CAD build for the part. Positions are in the model's coordinates, mm. A direction names the side the tool comes from. Coordinates: 2 decimals unless noted, no trailing zeros. Write each loop counter-clockwise with the first axis right and the second up, starting at its lowest first coordinate (ties: lowest second). Pieces come first, ordered by that corner, then holes. Notation, with made-up numbers: (-35, -36.75) - (0, -36.75) arc R36 ccw to (0, 2.25) - close; hole circle Ø8 at (65, -3). An arc over 180 degrees is marked (long way). Answer in a Markdown table with one row per item. Add a question column.
Q1. Band-saw the part on A-A (x = 0). List the corners of the cut face in (y, z) (3 decimals).
Q2. Two-plate mould, pull along Y, no slides. Class faces 4 (the cylindrical face through (-17.48, 6.86, 18.71)), 5 (the flat face through (18.75, -3, 20)), 6 (the cylindrical face through (-5.158, -3.955, -1.479)): +Y half, -Y half, draft (parallel to the pull), parting line (faces both ways), or undercut.
Q3. Drill centre lines: line 1 along X through (y, z) = (7, 16); line 2 along Z through (x, y) = (5, -8.5); line 3 along Y through (x, z) = (-10, 2.5). Where is each one in solid material? Low to high. Write a range as from..to.
Q4. Pin check, flat tips, straight feed: pin 1 (1 mm diameter, centred on x = -15, z = 16, fed in from +Y); pin 2 (9.5 mm diameter, centred on y = 0, z = 15.25, fed in from +X); pin 3 (0.8 mm diameter, centred on x = -15.5, y = -10.5, fed in from +Z). Stop position of each tip, or through.
Q5. Band-saw the part on C-C (y = -9.5). List the corners of the cut face in (x, z), and give its area (3 significant figures).
Q6. Band-saw the part on B-B (z = 6). List the corners of the cut face in (x, y), and give its area (4 significant figures).
Q7. Band-saw the part on D-D (z = 14.5). List the corners of the cut face in (x, y).
Q8. 3-axis set-ups, long thin cutter, end or side, ignore diameter. For faces 1 (the flat face through (-15.25, -1, 7)), 2 (the flat face through (17, 0, 35)), 3 (the flat face through (16, 6.981, 14)): which of +Z, -Z, +X, -X, +Y, -Y reach the whole face in a straight line?
```python
from build123d import *

# Parameters (mm, degrees)
SKETCH1_W            = 37.5
SKETCH1_H            = 24
SKETCH1_R            = 0.8
SKETCH1_R_2          = 6.5
BOSS_EXTRUDE1_DEPTH  = 3
SKETCH2_W            = 2.5
SKETCH2_H            = 40
BOSS_EXTRUDE2_DEPTH  = 24
BOSS_EXTRUDE3_DEPTH  = 1
BOSS_EXTRUDE4_START  = 31.5
BOSS_EXTRUDE4_DEPTH  = 1
M3_CLEARANCE_HOLE1_D = 3.6
CHAMFER1_SIZE        = 2
SKETCH7_R            = 3
SKETCH7_W            = 11
SKETCH7_H            = 9
CUT_EXTRUDE1_DEPTH   = 57.127087934
FILLET1_R            = 1
BOSS_EXTRUDE5_DEPTH  = 2
BOSS_EXTRUDE6_DEPTH  = 5


with BuildPart() as part:
    # Sketch1 → Boss-Extrude1 (new body)
    with BuildSketch(Plane.XY):
        Rectangle(SKETCH1_W, SKETCH1_H)
        with Locations((0, 9.075)):
            Circle(SKETCH1_R, mode=Mode.SUBTRACT)
        with Locations((7.859180539, -4.5375)):
            Circle(SKETCH1_R, mode=Mode.SUBTRACT)
        with Locations((-7.859180539, -4.5375)):
            Circle(SKETCH1_R, mode=Mode.SUBTRACT)
        Circle(SKETCH1_R_2, mode=Mode.SUBTRACT)
    extrude(amount=-BOSS_EXTRUDE1_DEPTH)

    # Sketch2 → Boss-Extrude2 (add)
    with BuildSketch(Plane(origin=(0, 12, 0), x_dir=(1, 0, 0), z_dir=(0, 1, 0))):
        with Locations((-17.5, -20)):
            Rectangle(SKETCH2_W, SKETCH2_H)
        with Locations((17.5, -20)):
            Rectangle(SKETCH2_W, SKETCH2_H)
    extrude(amount=-BOSS_EXTRUDE2_DEPTH)

    # Sketch4 → Boss-Extrude3 (add)
    with BuildSketch(Plane(origin=(-16.25, 0, 0), x_dir=(0, 0, -1), z_dir=(1, 0, 0))):
        with BuildLine():
            Line((-9.328443352, 3.861127794), (-9.37974654, -3.938739946))
            ThreePointArc((-9.37974654, -3.938739946), (-10.302425145, -6.124404492), (-12.500032536, -7.018265261))
            Line((-12.500032536, -7.018265261), (-15.407950321, -7.018265261))
            Line((-15.407950321, -7.018265261), (-15.407950321, -12))
            Line((-15.407950321, -12), (0, -12))
            Line((0, -12), (0, 12))
            Line((0, 12), (-15.407950321, 12))
            Line((-15.407950321, 12), (-15.407950321, 6.981431896))
            Line((-15.407950321, 6.981431896), (-12.407950321, 6.981431896))
            ThreePointArc((-12.407950321, 6.981431896), (-10.222291202, 6.058740436), (-9.328443352, 3.861127794))
        make_face()
    extrude(amount=BOSS_EXTRUDE3_DEPTH)

    # Sketch4<2> → Boss-Extrude4 (add)
    with BuildSketch(Plane(origin=(-16.25, 0, 0), x_dir=(0, 0, -1), z_dir=(1, 0, 0)).offset(BOSS_EXTRUDE4_START)):
        with BuildLine():
            Line((-9.328443352, 3.861127794), (-9.37974654, -3.938739946))
            ThreePointArc((-9.37974654, -3.938739946), (-10.302425145, -6.124404492), (-12.500032536, -7.018265261))
            Line((-12.500032536, -7.018265261), (-15.407950321, -7.018265261))
            Line((-15.407950321, -7.018265261), (-15.407950321, -12))
            Line((-15.407950321, -12), (0, -12))
            Line((0, -12), (0, 12))
            Line((0, 12), (-15.407950321, 12))
            Line((-15.407950321, 12), (-15.407950321, 6.981431896))
            Line((-15.407950321, 6.981431896), (-12.407950321, 6.981431896))
            ThreePointArc((-12.407950321, 6.981431896), (-10.222291202, 6.058740436), (-9.328443352, 3.861127794))
        make_face()
    extrude(amount=BOSS_EXTRUDE4_DEPTH)

    # M3 Clearance Hole1 (through all)
    with Locations(Plane(origin=(-18.75, 0, 0), x_dir=(0, 0, -1), z_dir=(-1, 0, 0))):
        with Locations((-20.599236057, 6.864991053), (-20.508469302, -6.934710444)):
            Hole(M3_CLEARANCE_HOLE1_D / 2)

    # Chamfer1
    chamfer1_edges = [part.edges().sort_by_distance(p)[0] for p in [
        (18.75, 0, -3),
        (-18.75, 0, -3),
        (-15.25, 0, 0),
        (15.25, 0, 0),
    ]]
    chamfer(chamfer1_edges, length=CHAMFER1_SIZE)

    # Sketch7 → Cut-Extrude1 (cut, through all)
    with BuildSketch(Plane.ZY.offset(18.75)):
        with Locations(Location((15.253967317, 7.63e-07, 0), (0, 0, 270))):
            Circle(SKETCH7_R)
        with Locations((29.5, 0)):
            Rectangle(SKETCH7_W, SKETCH7_H)
    extrude(amount=-CUT_EXTRUDE1_DEPTH, mode=Mode.SUBTRACT)

    # Fillet1
    fillet1_edges = [part.edges().sort_by_distance(p)[0] for p in [
        (-17.5, -4.5, 24),
        (-17.5, 4.5, 24),
        (-17.5, 4.5, 35),
        (-17.5, -4.5, 35),
        (17.5, -4.5, 24),
        (17.5, 4.5, 24),
        (17.5, 4.5, 35),
        (17.5, -4.5, 35),
    ]]
    fillet(fillet1_edges, radius=FILLET1_R)

    # Sketch8 → Boss-Extrude5 (add)
    with BuildSketch(Plane.XZ.offset(12)):
        Polygon((-16.75, -3), (16.75, -3), (18.75, -1), (18.75, 40), (16.25, 40), (16.25, 15.407950321), (15.25, 15.407950321), (15.25, 2), (13.25, 0), (-13.25, 0), (-15.25, 2), (-15.25, 15.407950321), (-16.25, 15.407950321), (-16.25, 40), (-18.75, 40), (-18.75, -1), align=None)
    extrude(amount=BOSS_EXTRUDE5_DEPTH)

    # Sketch9 → Boss-Extrude6 (add)
    with BuildSketch(Plane.XZ.offset(14)):
        Polygon((-18.75, 40), (18.75, 40), (18.75, -1), (16.75, -3), (-16.75, -3), (-18.75, -1), align=None)
    extrude(amount=BOSS_EXTRUDE6_DEPTH)


solid = part.part
```
Checked values:
| question | item | result |
|---|---|---|
| 1 | outline | (-19, -3) - (-6.5, -3) - (-6.5, 0) - (-14, 0) - (-14, 40) - (-19, 40) - close; (6.5, -3) - (8.275, -3) - (8.275, 0) - (6.5, 0) - close; (9.875, -3) - (12, -3) - (12, 0) - (9.875, 0) - close |
| 2 | face 4 | undercut |
| 2 | face 5 | draft |
| 2 | face 6 | undercut |
| 3 | line 1 | x = -18.75..-16.25, 16.25..18.75 |
| 3 | line 2 | z = -3..0 |
| 3 | line 3 | y = -19..-14 |
| 4 | pin 1 | stops at y = -14 |
| 4 | pin 2 | stops at x = 18.75 |
| 4 | pin 3 | stops at z = 15.41 |
| 5 | outline | (-18.75, -1) - (-16.75, -3) - (16.75, -3) - (18.75, -1) - (18.75, 40) - (16.25, 40) - (16.25, 15.41) - (15.25, 15.41) - (15.25, 2) - (13.25, 0) - (-13.25, 0) - (-15.25, 2) - (-15.25, 15.41) - (-16.25, 15.41) - (-16.25, 40) - (-18.75, 40) - close |
| 5 | area | 343 mm² |
| 6 | outline | (-18.75, -19) - (18.75, -19) - (18.75, 12) - (15.25, 12) - (15.25, -14) - (-15.25, -14) - (-15.25, 12) - (-18.75, 12) - close |
| 6 | area | 369.5 mm² |
| 7 | outline | (-18.75, -19) - (18.75, -19) - (18.75, -2.9) - (16.25, -2.9) - (16.25, -7.02) - (15.25, -7.02) - (15.25, -14) - (-15.25, -14) - (-15.25, -7.02) - (-16.25, -7.02) - (-16.25, -2.9) - (-18.75, -2.9) - close; (-18.75, 2.9) - (-16.25, 2.9) - (-16.25, 6.98) - (-15.25, 6.98) - (-15.25, 12) - (-18.75, 12) - close; (15.25, 6.98) - (16.25, 6.98) - (16.25, 2.9) - (18.75, 2.9) - (18.75, 12) - (15.25, 12) - close |
| 8 | face 1 | +Z, +Y |
| 8 | face 2 | +X, -X |
| 8 | face 3 | +Z |
